```python
from build123d import *

# Parameters (mm, degrees)
SKETCH1_W               = 180
SKETCH1_H               = 200
BOSS_EXTRUDE1_DEPTH     = 3
SKETCH2_W               = 180
SKETCH2_H               = 200
SKETCH2_W_2             = 176
SKETCH2_H_2             = 196
BOSS_EXTRUDE2_DEPTH     = 50
CUT_EXTRUDE1_DEPTH      = 145.599446749
CUT_EXTRUDE1_DEPTH_BACK = 145.599446749
SKETCH3_W               = 34.985098544
SKETCH3_H               = 34.434974118


with BuildPart() as part:
    # Sketch1 → Boss-Extrude1 (new body)
    with BuildSketch(Plane(origin=(0, 0, 0), x_dir=(1, 0, 0), z_dir=(0, 1, 0))):
        Rectangle(SKETCH1_W, SKETCH1_H)
    extrude(amount=BOSS_EXTRUDE1_DEPTH)

    # Sketch2 → Boss-Extrude2 (add)
    with BuildSketch(Plane(origin=(0, 3, 0), x_dir=(1, 0, 0), z_dir=(0, 1, 0))):
        Rectangle(SKETCH2_W, SKETCH2_H)
        Rectangle(SKETCH2_W_2, SKETCH2_H_2, mode=Mode.SUBTRACT)
    extrude(amount=BOSS_EXTRUDE2_DEPTH)

    # Sketch3 → Cut-Extrude1 (cut, two sides: drawn at the far end of the back side and taken through both)
    with BuildSketch(Plane.XY.offset(-CUT_EXTRUDE1_DEPTH_BACK)):
        with Locations((-50, 19.417487059)):
            Rectangle(SKETCH3_W, SKETCH3_H)
        with Locations((50, 19.417487059)):
            Rectangle(SKETCH3_W, SKETCH3_H)
    extrude(amount=CUT_EXTRUDE1_DEPTH + CUT_EXTRUDE1_DEPTH_BACK, mode=Mode.SUBTRACT)


solid = part.part
```
CAD build for the part. Positions are in the model's coordinates, mm. A direction names the side the tool comes from. Round coordinates to 2 decimals unless told otherwise and drop trailing zeros. Order: outer loops, then holes, each group sorted by start corner. A loop starts at its lowest first (then second) coordinate and runs counter-clockwise, first axis right, second up. Notation, with made-up numbers: (75.25, 21.25) -> (109.25, 21.25) arc R18 ccw to (109.25, 35.25) -> close; hole circle Ø10 at (53.25, -23). An arc over 180 degrees is marked (long way). One line per question, with ' | ' between items.
Q1. Which spindle directions (+Z, -Z, +X, -X, +Y, -Y) get a long thin tool onto all of the face, cutting with end or side? Do faces 5 (the flat face through (-1, 32, 100)), 6 (the flat face through (88, 28, 1)). Say none if no direction does.
Completed:
face 5: +Z, +X, -X, +Y, -Y | face 6: +Y
Q2. Slice it at C-C (z = 45). Write the cut outline in (x, y), then the cut area to 3 significant figures.
Completed:
outline: (-90, 0) -> (90, 0) -> (90, 53) -> (88, 53) -> (88, 3) -> (67.49, 3) -> (67.49, 2.2) -> (32.51, 2.2) -> (32.51, 3) -> (-32.51, 3) -> (-32.51, 2.2) -> (-67.49, 2.2) -> (-67.49, 3) -> (-88, 3) -> (-88, 53) -> (-90, 53) -> close | area: 684 mm^2
Q3. Slice it at A-A (y = 32). Write the cut outline in (x, z), then the cut area to 3 significant figures.
Completed:
outline: (-90, -100) -> (-67.49, -100) -> (-67.49, -98) -> (-88, -98) -> (-88, 98) -> (-67.49, 98) -> (-67.49, 100) -> (-90, 100) -> close; (-32.51, -100) -> (32.51, -100) -> (32.51, -98) -> (-32.51, -98) -> close; (-32.51, 98) -> (32.51, 98) -> (32.51, 100) -> (-32.51, 100) -> close; (67.49, -100) -> (90, -100) -> (90, 100) -> (67.49, 100) -> (67.49, 98) -> (88, 98) -> (88, -98) -> (67.49, -98) -> close | area: 1,220 mm^2
Q4. Probe probe 1 along X at (y, z) = (6.5, 4.5); probe 2 along Z at (x, y) = (-20, 39); probe 3 along Y at (x, z) = (-6, -42.5). List the from-to ranges inside material, lowest first.
Completed:
probe 1: x = -90 to -88, 88 to 90 | probe 2: z = -100 to -98, 98 to 100 | probe 3: y = 0 to 3
Q5. Drop flat-ended pins along their axis: pin 1 (8 mm diameter, centred on x = -66, y = 31.5, fed in from -Z); pin 2 (17.5 mm diameter, centred on x = 51, z = 15.5, fed in from +Y); pin 3 (10.5 mm diameter, centred on x = 80.5, z = 26, fed in from +Y). Give the stop position or say it passes through.
Completed:
pin 1: stops at z = -100 | pin 2: stops at y = 2.2 | pin 3: stops at y = 3
Q6. Slice it at B-B (x = 64). Write the cut outline in (y, z).
Completed:
outline: (0, -100) -> (2.2, -100) -> (2.2, 100) -> (0, 100) -> close; (36.63, -100) -> (53, -100) -> (53, -98) -> (36.63, -98) -> close; (36.63, 98) -> (53, 98) -> (53, 100) -> (36.63, 100) -> close
Q7. Slice it at D-D (y = 49.5). Write the cut outline in (x, z).
Completed:
outline: (-90, -100) -> (90, -100) -> (90, 100) -> (-90, 100) -> close; hole (-88, -98) -> (88, -98) -> (88, 98) -> (-88, 98) -> close
Q8. Two-plate mould, pull along X, no slides. Class faces 1 (the flat face through (-1, 33, -98)), 2 (the flat face through (-90, 26, 1)), 3 (the flat face through (-1, 0, -1)), 4 (the flat face through (90, 26, 1)): released by +X, released by -X, zero draft, split by the parting line, or undercut.
Completed:
face 1: undercut | face 2: released by -X | face 3: zero draft | face 4: released by +X
